Autodesk Inventor part; units mm, degrees
ref_plane "YZ Plane" through (0, 0, 0) normal (1, 0, 0) x (0, 1, 0)
ref_plane "XZ Plane" through (0, 0, 0) normal (0, 1, 0) x (-1, 0, 0)
ref_plane "XY Plane" through (0, 0, 0) normal (0, 0, 1) x (1, 0, 0)
sketch "main" plane through (0, 0, 0) normal (0, 0, 1) x (1, 0, 0)
  line L0 (-25.7346, 15.6158) -> (-23.1842, 13.0654)
  arc A0 (-23.1842, 12.347) -> (-23.1842, 13.0654) centre (-23.5434, 12.7062) ccw
  line L1 (-23.1842, 12.347) -> (-25.7346, 9.7966)
  line L2 (-29.0034, 13.0654) -> (-26.453, 15.6158)
  circle A1 centre (-26.0938, 12.7062) radius 2.1844 construction
  arc A2 (-29.0034, 13.0654) -> (-29.0034, 12.347) centre (-28.6442, 12.7062) ccw
  line L3 (-26.453, 9.7966) -> (-29.0034, 12.347)
  arc A3 (-32.1645, 3.3667) -> (-32.1645, 4.0851) centre (-32.5237, 3.7259) ccw
  arc A4 (-26.453, 9.7966) -> (-25.7346, 9.7966) centre (-26.0938, 10.1558) ccw
  arc A5 (-8.6781, 35.1568) -> (-15.4133, 32.367) centre (-8.6781, 25.6318) ccw
  circle A6 centre (-17.1136, 21.6864) radius 2.1844
  arc A7 (-25.7346, 15.6158) -> (-26.453, 15.6158) centre (-26.0938, 15.2566) ccw
  line L4 (-10.1527, 19.667) -> (-30.584, -0.7642)
  line L5 (-39.5642, 8.216) -> (-15.4133, 32.367)
  line L6 (-17.1136, 21.6864) -> (-10.7636, 21.6864) construction
  line L7 (-17.1136, 21.6864) -> (-21.6037, 26.1765)
  arc A8 (-34.7149, 6.6355) -> (-35.4333, 6.6355) centre (-35.0741, 6.2763) ccw
  line L8 (-34.7149, 6.6355) -> (-32.1645, 4.0851)
  line L9 (-32.1645, 3.3667) -> (-34.7149, 0.8163)
  arc A9 (-37.9837, 4.0851) -> (-37.9837, 3.3667) centre (-37.6245, 3.7259) ccw
  arc A10 (-35.4333, 0.8163) -> (-34.7149, 0.8163) centre (-35.0741, 1.1755) ccw
  line L10 (-35.4333, 0.8163) -> (-37.9837, 3.3667)
  arc A11 (-39.5642, 8.216) -> (-30.584, -0.7642) centre (-35.0741, 3.7259) ccw
  line L11 (-37.9837, 4.0851) -> (-35.4333, 6.6355)
  circle A12 centre (43.5032, -3.0093) radius 2.1844
  circle A13 centre (25.5426, -20.9698) radius 2.1844
  arc A14 (21.0525, -16.4797) -> (30.0328, -25.4599) centre (25.5426, -20.9698) ccw
  line L12 (21.0525, -16.4797) -> (40.6569, 3.1247)
  line L13 (50.966, -4.5267) -> (30.0328, -25.4599)
  circle A15 centre (59.4482, 5.5431) radius 2.1844
  line L14 (72.1482, 11.8931) -> (63.3936, 11.8931)
  line L15 (56.6584, 14.6829) -> (38.9743, 32.367)
  line L16 (72.1482, -0.8069) -> (59.9463, -0.8069)
  arc A16 (56.6584, 14.6829) -> (63.3936, 11.8931) centre (63.3936, 21.4181) ccw
  line L17 (84.8482, 11.8931) -> (72.1482, 11.8931)
  line L18 (84.8482, -0.8069) -> (72.1482, -0.8069)
  circle A17 centre (84.8482, 5.5431) radius 2.1844
  arc A18 (84.8482, -0.8069) -> (84.8482, 11.8931) centre (84.8482, 5.5431) ccw
  arc A19 (59.9463, -0.8069) -> (50.966, -4.5267) centre (59.9463, -13.5069) ccw
  arc A20 (-3.4175, 22.4568) -> (-10.1527, 19.667) centre (-3.4175, 12.9318) ccw
  line L19 (-3.4175, 22.4568) -> (28.3325, 22.4568)
  line L20 (-8.6781, 35.1568) -> (32.2391, 35.1568)
  arc A21 (31.7001, 21.0619) -> (28.3325, 22.4568) centre (28.3325, 17.6943) ccw
  arc A22 (38.9743, 32.367) -> (32.2391, 35.1568) centre (32.2391, 25.6318) ccw
  line L21 (31.7001, 21.0619) -> (40.6569, 12.105)
  line L22 (31.7001, 21.0619) -> (44.367, 21.0619) construction
  arc A23 (40.6569, 3.1247) -> (40.6569, 12.105) centre (36.1668, 7.6149) ccw
  circle A24 centre (25.1575, 28.8068) radius 2.1844
  circle A25 centre (-0.2425, 28.8068) radius 2.1844
  point P0 (7.2046, 10.3806)
  point P1 (59.4482, 11.8931)
  dimension "d5" = 12.7
  dimension "d6" = 135
  dimension "d7" = 9.525
  dimension "d8" = 12.7
  dimension "d9" = 9.525
  dimension "d10" = 9.525
  dimension "d11" = 12.7
  dimension "d12" = 4.7625
  dimension "d15" = 31.75
  dimension "d16" = 12.7
  dimension "d17" = 45
  dimension "d18" = 6.35
  dimension "d19" = 4.3688
  dimension "d20" = 6.35
  dimension "d24" = 4.3688
sketch "Sketch1" plane through (0, 0, 0) normal (0, 1, 0) x (-1, 0, 0)
  line L0 (-85.1829, 10.0727) -> (-82.6325, 7.5223)
  arc A0 (-82.6325, 6.8039) -> (-82.6325, 7.5223) centre (-82.9917, 7.1631) ccw
  line L1 (-82.6325, 6.8039) -> (-85.1829, 4.2535)
  line L2 (-88.4517, 7.5223) -> (-85.9013, 10.0727)
  circle A1 centre (-85.5421, 7.1631) radius 2.1844 construction
  arc A2 (-88.4517, 7.5223) -> (-88.4517, 6.8039) centre (-88.0925, 7.1631) ccw
  line L3 (-85.9013, 4.2535) -> (-88.4517, 6.8039)
  arc A3 (-91.6127, -2.1764) -> (-91.6127, -1.4579) centre (-91.9719, -1.8171) ccw
  arc A4 (-85.9013, 4.2535) -> (-85.1829, 4.2535) centre (-85.5421, 4.6127) ccw
  arc A5 (-68.1263, 29.6137) -> (-74.8615, 26.8239) centre (-68.1263, 20.0887) ccw
  circle A6 centre (-76.5618, 16.1434) radius 2.1844
  arc A7 (-85.1829, 10.0727) -> (-85.9013, 10.0727) centre (-85.5421, 9.7135) ccw
  line L4 (-69.601, 14.1239) -> (-90.0322, -6.3073)
  line L5 (-99.0125, 2.673) -> (-74.8615, 26.8239)
  line L6 (-76.5618, 16.1434) -> (-70.2118, 16.1434) construction
  line L7 (-76.5618, 16.1434) -> (-81.0519, 20.6335)
  arc A8 (-94.1631, 1.0925) -> (-94.8815, 1.0925) centre (-94.5223, 0.7332) ccw
  line L8 (-94.1631, 1.0925) -> (-91.6127, -1.4579)
  line L9 (-91.6127, -2.1764) -> (-94.1631, -4.7268)
  arc A9 (-97.4319, -1.4579) -> (-97.4319, -2.1764) centre (-97.0727, -1.8171) ccw
  arc A10 (-94.8815, -4.7268) -> (-94.1631, -4.7268) centre (-94.5223, -4.3675) ccw
  line L10 (-94.8815, -4.7268) -> (-97.4319, -2.1764)
  arc A11 (-99.0125, 2.673) -> (-90.0322, -6.3073) centre (-94.5223, -1.8172) ccw
  line L11 (-97.4319, -1.4579) -> (-94.8815, 1.0925)
  circle A12 centre (-15.9451, -8.5524) radius 2.1844
  circle A13 centre (-33.9056, -26.5129) radius 2.1844
  arc A14 (-38.3957, -22.0227) -> (-29.4155, -31.003) centre (-33.9056, -26.5129) ccw
  line L12 (-38.3957, -22.0227) -> (-18.7913, -2.4183)
  line L13 (-8.4822, -10.0697) -> (-29.4155, -31.003)
  circle A15 centre (0, 0) radius 2.1844
  line L14 (12.7, 6.35) -> (3.9454, 6.35)
  line L15 (-2.7898, 9.1398) -> (-20.4739, 26.8239)
  line L16 (12.7, -6.35) -> (0.498, -6.35)
  arc A16 (-2.7898, 9.1398) -> (3.9454, 6.35) centre (3.9454, 15.875) ccw
  line L17 (25.4, 6.35) -> (12.7, 6.35)
  line L18 (25.4, -6.35) -> (12.7, -6.35)
  circle A17 centre (25.4, 0) radius 2.1844
  arc A18 (25.4, -6.35) -> (25.4, 6.35) centre (25.4, 0) ccw
  arc A19 (0.498, -6.35) -> (-8.4822, -10.0697) centre (0.498, -19.05) ccw
  arc A20 (-62.8658, 16.9137) -> (-69.601, 14.1239) centre (-62.8658, 7.3887) ccw
  line L19 (-62.8658, 16.9137) -> (-31.1158, 16.9137)
  line L20 (-68.1263, 29.6137) -> (-27.2091, 29.6137)
  arc A21 (-27.7482, 15.5188) -> (-31.1158, 16.9137) centre (-31.1158, 12.1512) ccw
  arc A22 (-20.4739, 26.8239) -> (-27.2091, 29.6137) centre (-27.2091, 20.0887) ccw
  line L21 (-27.7482, 15.5188) -> (-18.7913, 6.5619)
  line L22 (-27.7482, 15.5188) -> (-15.0812, 15.5188) construction
  arc A23 (-18.7913, -2.4183) -> (-18.7913, 6.5619) centre (-23.2814, 2.0718) ccw
  circle A24 centre (-34.2908, 23.2637) radius 2.1844
  circle A25 centre (-59.6908, 23.2637) radius 2.1844
extrude "Extrusion1" add sketch "Sketch1" along normal blind 1.5875
properties part number "join_gusset" material "Acetal Resin, White"
Source: CAD feature listing. Evaluate the final solid. Frame: model axes, mm. A direction names the side the tool comes from. Coordinates: 2 decimals unless noted, no trailing zeros. Loops run counter-clockwise (first coordinate to the right, second up) from the corner with the lowest first, then second, coordinate; pieces in that order, holes last. Notation, with made-up numbers: M 27.5,-4.75 L 33.5,-4.75 A23 ccw 33.5,27.25 Z; hole C 67,2.5 d9. An arc over 180 degrees is marked long. Put each result on its own line as item: value. Start each with the question number.
1) Ray query, L1, parallel to X at y = 0.75, z = 8; L2, parallel to X at y = 1.05, z = 22; L3, parallel to Z at x = 60, y = 0.95. Return the intervals inside material, ascending. Write a range as from..to.
2) Cut plane B-B on y = 1.2. Give the number of separate pieces and of enclosed holes in the cut face, then the cut area to 3 significant figures.
3) Cut plane A-A on x = -21. Return the cut outline in (y, z).
4) Contact query for flat-ended pins moving along their axis: pin 1 Ø4 at (x, z) = (-25.4, 0) entering from +Y; pin 2 Ø0.8 at (x, y) = (-17.5, 1) entering from +Z. Output: stop coordinate, or through.
5) Pull-direction query (Z, two-part tool) for faces 3 (the face through (98.91, 0.78, -6.41)), 4 (the face through (35.639, 0.783, -25.184)), 5 (the face through (-0.349, 0.783, 7.055)); classes: pulls with the +Z half, pulls with the -Z half, needs draft (parallel to the pull), parting line crosses it, or undercut.
6) Reachability of faces 1 (the face through (96.14, 0.78, -3.47)), 2 (the face through (30, 0, 19)) from +Z, -Z, +X, -X, +Y, -Y: full face, straight path, thin tool, end or side. Return the list, or none.
The answers:
1. L1: x = 1.41..20.23, 75.72..83.11, 87.97..93.69
1. L2: x = 15.65..32.51, 36.07..57.91, 61.47..79.69
1. L3: z = 16.91..21.1, 25.43..29.61
2. separate pieces: 1
2. enclosed holes: 9
2. area: 2,280 mm²
3. outline: M 0,-6.35 L 1.59,-6.35 L 1.59,6.35 L 0,6.35 Z
4. pin 1: passes through
4. pin 2: stops at z = 6.35
5. face 3: parting line crosses it
5. face 4: undercut
5. face 5: pulls with the +Z half
6. face 1: +Y, -Y
6. face 2: +Z, -Z, +X, -X, -Y
